from build123d import *

# Parameters (mm, degrees)
SKETCH1_W           = 85
SKETCH1_H           = 85
BOSS_EXTRUDE1_DEPTH = 32
SKETCH2_R           = 3
CUT_EXTRUDE1_DEPTH  = 33
SKETCH3_R           = 5
SKETCH3_R_2         = 6
CUT_EXTRUDE2_DEPTH  = 86
SKETCH4_R           = 3
CUT_EXTRUDE3_DEPTH  = 33


with BuildPart() as part:
    # Sketch1 → Boss-Extrude1 (new body)
    with BuildSketch(Plane.XY):
        Rectangle(SKETCH1_W, SKETCH1_H)
    extrude(amount=BOSS_EXTRUDE1_DEPTH)

    # Sketch2 → Cut-Extrude1 (cut, through all)
    with BuildSketch(Plane.XY.offset(32)):
        with Locations((-36.5, 36.5)):
            Circle(SKETCH2_R)
        with Locations((36.5, 36.5)):
            Circle(SKETCH2_R)
        with Locations((36.5, -36.5)):
            Circle(SKETCH2_R)
        with Locations((-36.5, -36.5)):
            Circle(SKETCH2_R)
    extrude(amount=-CUT_EXTRUDE1_DEPTH, mode=Mode.SUBTRACT)

    # Sketch3 → Cut-Extrude2 (cut, through all)
    with BuildSketch(Plane(origin=(0, 42.5, 0), x_dir=(1, 0, 0), z_dir=(0, 1, 0))):
        with Locations((0, -16)):
            Circle(SKETCH3_R)
        with Locations((-23, -16)):
            Circle(SKETCH3_R_2)
        with Locations((23, -16)):
            Circle(SKETCH3_R_2)
    extrude(amount=-CUT_EXTRUDE2_DEPTH, mode=Mode.SUBTRACT)

    # Sketch4 → Cut-Extrude3 (cut, through all)
    with BuildSketch(Plane(origin=(0, 0, 0), x_dir=(-1, 0, 0), z_dir=(0, 0, -1))):
        with Locations((-35.5, 18)):
            Circle(SKETCH4_R)
        with Locations((-35.5, -18)):
            Circle(SKETCH4_R)
        with Locations((35.5, -18)):
            Circle(SKETCH4_R)
        with Locations((35.5, 18)):
            Circle(SKETCH4_R)
    extrude(amount=-CUT_EXTRUDE3_DEPTH, mode=Mode.SUBTRACT)


solid = part.part
Can you work these out from the model? Positions are in its coordinate system, mm. Coordinates: 2 decimals unless noted, no trailing zeros. Write each loop counter-clockwise with the first axis right and the second up, starting at its lowest first coordinate (ties: lowest second). Pieces come first, ordered by that corner, then holes.
Q1. If we mould it in two halves opening along Y, with no side actions, what happens to faces 1 (the face through (-38.71, 38.53, 16.22)), 2 (the face through (-1, 42.5, 9)), 3 (the face through (42.5, -1, 16)), 4 (the face through (-1, -42.5, 9))? For each: +Y half, -Y half, draft (parallel to the pull), parting line (faces both ways), or undercut.
Results found:
face 1: undercut
face 2: +Y half
face 3: draft
face 4: -Y half
Q2. For P1, Ø8, axis at x = 0, z = 16, coming from the +Y side; P2, Ø6, axis at x = 2.5, y = -17, coming from the -Z side, each with a flat end and sliding along its axis, tell me the tip position at first contact or that it passes through.
Results found:
P1: passes through
P2: stops at z = 0
Q3. Imagine slicing it at B-B, the plane z = 16. Count the separate pieces of the cut face and the enclosed holes in it, plus the area to 3 significant figures.
Results found:
separate pieces: 4
enclosed holes: 8
area: 4,110 mm2
Q4. Imagine slicing it at C-C, the plane x = -23. List the corners of the cut face in (y, z) for me.
Results found:
outline: (-42.5, 0) - (42.5, 0) - (42.5, 10) - (-42.5, 10) - close; (-42.5, 22) - (42.5, 22) - (42.5, 32) - (-42.5, 32) - close
Q5. Imagine slicing it at A-A, the plane y = 18. List the corners of the cut face in (x, z) for me, plus the area to 3 significant figures.
Results found:
outline: (-42.5, 0) - (-38.5, 0) - (-38.5, 32) - (-42.5, 32) - close; (-32.5, 0) - (32.5, 0) - (32.5, 32) - (-32.5, 32) - close; (38.5, 0) - (42.5, 0) - (42.5, 32) - (38.5, 32) - close; hole circle Ø12 at (-23, 16); hole circle Ø10 at (0, 16); hole circle Ø12 at (23, 16)
area: 2,030 mm2
Q6. Please list where these lines run through material, in increasing order: L1, parallel to X at y = 4, z = 16; L2, parallel to Z at x = 23, y = 5; L3, parallel to Y at x = 35, z = 21.5.
Results found:
L1: x = -42.5 to -29, -17 to -5, 5 to 17, 29 to 42.5
L2: z = 0 to 10, 22 to 32
L3: y = -42.5 to -39.1, -33.9 to -20.96, -15.04 to 15.04, 20.96 to 33.9, 39.1 to 42.5
